Could you check a few things on this model? Use its own coordinates, in mm. A direction names the side the tool comes from. Give positions to 0.01 mm unless a question says otherwise; leave off trailing zeros. Loops run counter-clockwise (first coordinate to the right, second up) from the corner with the lowest first, then second, coordinate; pieces in that order, holes last. Notation, with made-up numbers: M -18.75,65.25 L 0.25,65.25 A20 cw 0.25,101.25 Z; hole C 74.25,11 d3. An arc over 180 degrees is marked long. Answer in a Markdown table with one row per item. Add a question column.
1. Thinking about a two-plate mould opening in X: for faces 4 (the flat face through (6, 13.093, 1)), 5 (the cylindrical face through (17.83, -4.22, 1.48)), 6 (the flat face through (6, 3.843, -9)), 7 (the flat face through (20.563, -3, 1)), which applies, released by +X, released by -X, zero draft, split by the parting line, or undercut?
2. Which directions (+Z, -Z, +X, -X, +Y, -Y) give clear straight access to the entire face, cutting with the end or side of a thin tool? Please do faces 1 (the cylindrical face through (13.91, -16.82, 1.62)), 2 (the flat face through (6, -10.157, -9)), 3 (the flat face through (-51.937, 8, 1)).
3. I need wall thicknesses on line 1 along X through (y, z) = (-10.95, -7); line 2 along X through (y, z) = (-2, 0.5); line 3 along X through (y, z) = (-15, 2.25). Which ranges of each line are inside material? Lowest first, please. Write a range as from..to.
4. If we section it at B-B on z = -1.5: List the corners of the cut face in (x, y) for me.
5. I'm going to push flat-ended pins straight in: pin 1 Ø1.4 at (y, z) = (-12.5, -3.5) entering from -X; pin 2 Ø2 at (x, y) = (-6.44, -18.66) entering from +Z; pin 3 Ø12 at (x, y) = (-12.5, 0) entering from -Z; pin 4 Ø3.5 at (y, z) = (-10, -6) entering from +X. Where does each tip first touch, or does it pass through?
6. If we section it at C-C on x = -19: List the corners of the cut face in (y, z) for me, then the cut area to 3 significant figures.
7. If we section it at D-D on z = -6: List the corners of the cut face in (x, y) for me, then the cut area to 3 significant figures.
8. If we section it at A-A on y = 6: Count the separate pieces of the cut face and the enclosed holes in it, then the cut area to 3 significant figures.
```python
from build123d import *

# Parameters (mm, degrees)
SKETCH1_W           = 65
SKETCH1_H           = 45
BOSS_EXTRUDE1_DEPTH = 3
FILLET4_R           = 10
BOSS_EXTRUDE4_DEPTH = 3
SKETCH9_R           = 1.75
CUT_EXTRUDE5_DEPTH  = 5
SKETCH10_R          = 1.75
SKETCH10_R_2        = 11.5
CUT_EXTRUDE6_DEPTH  = 5
SKETCH2_W           = 10
SKETCH2_H           = 4
BOSS_EXTRUDE5_DEPTH = 12
SKETCH11_R          = 1.75
CUT_EXTRUDE7_DEPTH  = 22
CHAMFER3_SIZE       = 2.5
CHAMFER4_SIZE       = 5
FILLET5_R           = 5
SKETCH13_W          = 12
SKETCH13_H          = 5.25


with BuildPart() as part:
    # Sketch1 → Boss-Extrude1 (new body)
    with BuildSketch(Plane.XY):
        with Locations((-11.936997319, -3.156836461)):
            Rectangle(SKETCH1_W, SKETCH1_H)
    extrude(amount=BOSS_EXTRUDE1_DEPTH)

    # Fillet4
    fillet4_edges = [part.edges().sort_by_distance(p)[0] for p in [
        (20.563002681, 19.343163539, 1.5),
        (20.563002681, -25.656836461, 1.5),
    ]]
    fillet(fillet4_edges, radius=FILLET4_R)

    # Sketch8 → Boss-Extrude4 (add)
    with BuildSketch(Plane(origin=(0, 0, 0), x_dir=(-1, 0, 0), z_dir=(0, 0, -1))):
        Polygon((44.436997319, 6.843163539), (51.936997319, 6.843163539), (51.936997319, 9.343163539), (59.436997319, 4.091607002), (59.436997319, -10.405279925), (51.936997319, -15.656836461), (51.936997319, -13.156836461), (44.436997319, -13.156836461), align=None)
    extrude(amount=-BOSS_EXTRUDE4_DEPTH)

    # Sketch9 → Cut-Extrude5 (cut)
    with BuildSketch(Plane(origin=(0, 0, 0), x_dir=(-1, 0, 0), z_dir=(0, 0, -1))):
        with Locations((-16.440039295, -3.156836461)):
            Circle(SKETCH9_R)
        with Locations((-3.563002681, -22.656836461)):
            Circle(SKETCH9_R)
        with Locations((41.436997319, -22.656836461)):
            Circle(SKETCH9_R)
        with Locations(Location((41.436997319, 16.343163539, 0), (0, 0, 180))):
            Circle(SKETCH9_R)
        with Locations(Location((-3.563002681, 16.343163539, 0), (0, 0, 180))):
            Circle(SKETCH9_R)
    extrude(amount=-CUT_EXTRUDE5_DEPTH, mode=Mode.SUBTRACT)

    # Sketch10 → Cut-Extrude6 (cut)
    with BuildSketch(Plane(origin=(0, 0, 0), x_dir=(-1, 0, 0), z_dir=(0, 0, -1))):
        with Locations((6.436997319, -18.656836461)):
            Circle(SKETCH10_R)
        with Locations((37.436997319, 12.343163539)):
            Circle(SKETCH10_R)
        with Locations((6.436997319, 12.343163539)):
            Circle(SKETCH10_R)
        with Locations((37.436997319, -18.656836461)):
            Circle(SKETCH10_R)
        with Locations((21.936997319, -3.156836461)):
            Circle(SKETCH10_R_2)
    extrude(amount=-CUT_EXTRUDE6_DEPTH, mode=Mode.SUBTRACT)

    # Sketch2 → Boss-Extrude5 (add)
    with BuildSketch(Plane(origin=(0, 0, 0), x_dir=(-1, 0, 0), z_dir=(0, 0, -1))):
        with Locations((-5.563002681, 5.843163539)):
            Rectangle(SKETCH2_W, SKETCH2_H)
        with Locations((-5.563002681, -12.156836461)):
            Rectangle(SKETCH2_W, SKETCH2_H)
    extrude(amount=BOSS_EXTRUDE5_DEPTH)

    # Sketch11 → Cut-Extrude7 (cut)
    with BuildSketch(Plane.XZ.offset(14.156836461)):
        with Locations(Location((5.563002681, -7, 0), (0, 0, 270))):
            Circle(SKETCH11_R)
    extrude(amount=-CUT_EXTRUDE7_DEPTH, mode=Mode.SUBTRACT)

    # Chamfer3
    chamfer3_edges = [part.edges().sort_by_distance(p)[0] for p in [
        (10.563002681, -12.156836461, 0),
        (0.563002681, -12.156836461, 0),
        (0.563002681, 5.843163539, 0),
        (10.563002681, 5.843163539, 0),
    ]]
    chamfer(chamfer3_edges, length=CHAMFER3_SIZE)

    # Chamfer4
    chamfer4_edges = [part.edges().sort_by_distance(p)[0] for p in [
        (5.563002681, -10.156836461, 0),
        (5.563002681, 3.843163539, 0),
    ]]
    chamfer(chamfer4_edges, length=CHAMFER4_SIZE)

    # Fillet5
    fillet5_edges = [part.edges().sort_by_distance(p)[0] for p in [
        (0.563002681, -12.156836461, -12),
        (10.563002681, -12.156836461, -12),
        (0.563002681, 5.843163539, -12),
        (10.563002681, 5.843163539, -12),
    ]]
    fillet(fillet5_edges, radius=FILLET5_R - 0.0001)  # a hair under: the kernel refuses the full size

    # Sketch13 → Cut-Revolve1 (revolve, cut)
    with BuildSketch(Plane(origin=(5.563002681, 0, 0), x_dir=(0, 0, -1), z_dir=(1, 0, 0))):
        with Locations((13, 10.468163539)):
            Rectangle(SKETCH13_W, SKETCH13_H)
    cut_revolve1 = revolve(axis=Axis((5.563002681, 7.843163539, -7), (0, -1, 0)), mode=Mode.SUBTRACT)

    # Mirror1: Cut-Revolve1 across plane
    add(cut_revolve1.mirror(Plane.ZX.offset(-3.156836461)), mode=Mode.SUBTRACT)


solid = part.part
```
Results:
| question | item | result |
|---|---|---|
| 1 | face 4 | undercut |
| 1 | face 5 | undercut |
| 1 | face 6 | zero draft |
| 1 | face 7 | released by +X |
| 2 | face 1 | -Z |
| 2 | face 2 | -Z, +X, -X |
| 2 | face 3 | +Z, -Z, +Y |
| 3 | line 1 | 0.56..3.81, 7.31..10.56 |
| 3 | line 2 | -59.44..-33.38, -10.5..15.13, 17.75..20.56 |
| 3 | line 3 | -52.88..-51.94, -44.44..-2.08, 13.21..20.56 |
| 4 | outline | M -0.44,-14.16 L 11.56,-14.16 L 11.56,-6.66 L -0.44,-6.66 Z; M -0.44,0.34 L 11.56,0.34 L 11.56,7.84 L -0.44,7.84 Z |
| 5 | pin 1 | x = 0.56 |
| 5 | pin 2 | through |
| 5 | pin 3 | z = 0 |
| 5 | pin 4 | x = 10.56 |
| 6 | outline | M -25.66,0 L -14.28,0 L -14.28,3 L -25.66,3 Z; M 7.96,0 L 19.34,0 L 19.34,3 L 7.96,3 Z |
| 6 | area | 68.3 mm2 |
| 7 | outline | M 0.56,-14.16 L 4.13,-14.16 L 4.13,-10.16 L 0.56,-10.16 Z; M 0.56,3.84 L 4.13,3.84 L 4.13,7.84 L 0.56,7.84 Z; M 7,-14.16 L 10.56,-14.16 L 10.56,-10.16 L 7,-10.16 Z; M 7,3.84 L 10.56,3.84 L 10.56,7.84 L 7,7.84 Z |
| 7 | area | 57.0 mm2 |
| 8 | separate pieces | 2 |
| 8 | enclosed holes | 1 |
| 8 | area | 296 mm2 |
